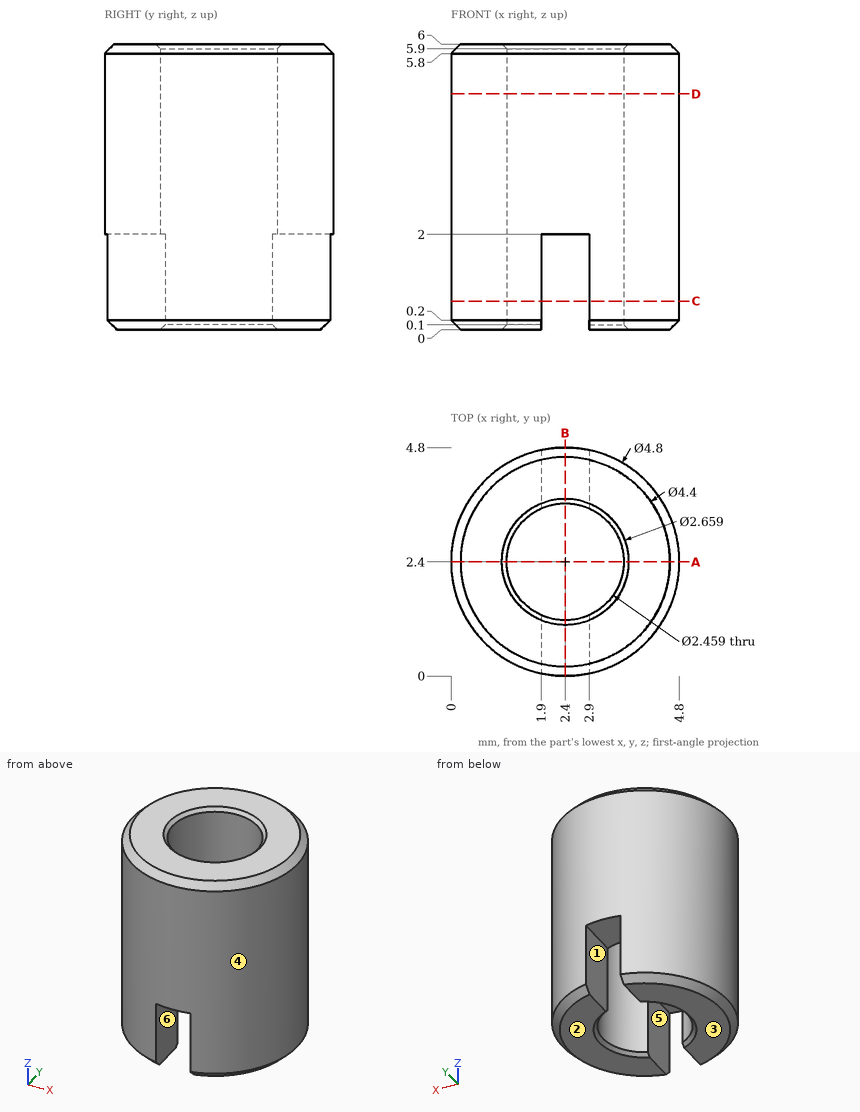
Could you check a few things on this drawing? It's one solid part, dimensions in mm from its lowest x, y, z. A direction names the side the tool comes from. Coordinates: 2 decimals unless noted, no trailing zeros. Order: outer loops, then holes, each group sorted by start corner. A loop starts at its lowest first (then second) coordinate and runs counter-clockwise, first axis right, second up. Notation, with made-up numbers: M 63,21 L 83,21 A27 ccw 83,38 Z; hole C 6,37.25 d4. An arc over 180 degrees is marked long. Use a Markdown table: item, result. Add a question column.
Q1. I want a section at D-D on z = 4.95. List the corners of the cut face in (x, y) for me, then the cut area to 3 significant figures.
Q2. I want a section at A-A on y = 2.4. List the corners of the cut face in (x, z) for me, then the cut area to 3 significant figures.
Q3. I'm going to push flat-ended pins straight in: pin 1 (1 mm diameter, centred on y = 0.5, z = 1.5, fed in from +X); pin 2 (1 mm diameter, centred on x = 3, z = 2.5, fed in from -Y); pin 3 (1 mm diameter, centred on y = 0.5, z = 1, fed in from -X). Where does each tip first touch, or does it pass through?
Q4. We'd pull the mould along X, two halves only. Please class the marked faces 3, 4, 5 and 6: pulls with the +X half, pulls with the -X half, needs draft (parallel to the pull), parting line crosses it, or undercut.
Q5. If I drill on L1, parallel to Y at x = 2.4, z = 4.1; L2, parallel to Y at x = 1.35, z = 3.35, over which ranges is the centre line in solid material (lowest first)?
Q6. I want a section at B-B on x = 2.4. List the corners of the cut face in (y, z) for me.
Q7. I want a section at C-C on z = 0.6. List the corners of the cut face in (x, y) for me.
Q8. Which directions (+Z, -Z, +X, -X, +Y, -Y) give clear straight access to the entire face, cutting with the end or side of a thin tool? Please do the marked faces 1 and 2.
Checked values:
| question | item | result |
|---|---|---|
| 1 | outline | C 2.4,2.4 d4.8; hole C 2.4,2.4 d2.46 |
| 1 | area | 13.3 mm² |
| 2 | outline | M 0,0.2 L 0.2,0 L 1.07,0 L 1.17,0.1 L 1.17,5.9 L 1.07,6 L 0.2,6 L 0,5.8 Z; M 3.63,0.1 L 3.73,0 L 4.6,0 L 4.8,0.2 L 4.8,5.8 L 4.6,6 L 3.73,6 L 3.63,5.9 Z |
| 2 | area | 13.9 mm² |
| 3 | pin 1 | x = 4.35 |
| 3 | pin 2 | y = 0 |
| 3 | pin 3 | x = 0.45 |
| 4 | face 3 | needs draft |
| 4 | face 4 | parting line crosses it |
| 4 | face 5 | undercut |
| 4 | face 6 | undercut |
| 5 | L1 | 0 to 1.17, 3.63 to 4.8 |
| 5 | L2 | 0.24 to 1.76, 3.04 to 4.56 |
| 6 | outline | M 0,2 L 1.17,2 L 1.17,5.9 L 1.07,6 L 0.2,6 L 0,5.8 Z; M 3.63,2 L 4.8,2 L 4.8,5.8 L 4.6,6 L 3.73,6 L 3.63,5.9 Z |
| 7 | outline | M 1.9,0.05 L 1.9,1.28 A1.23 cw 1.9,3.52 L 1.9,4.75 A2.4 ccw Z; M 2.9,0.05 A2.4 ccw 2.9,4.75 L 2.9,3.52 A1.23 cw 2.9,1.28 Z |
| 8 | face 1 | -Z, +Y, -Y |
| 8 | face 2 | -Z, +X, -X, +Y, -Y |
